The drawing under review shows one solid part. Ordinate dimensions are in mm from its lowest x, y, z. Give positions to 0.01 mm unless a question says otherwise; leave off trailing zeros. Order: outer loops, then holes, each group sorted by start corner. A loop starts at its lowest first (then second) coordinate and runs counter-clockwise, first axis right, second up. Notation, with made-up numbers: (-31.5, 80.25) -> (-3.5, 80.25) arc R12 cw to (-3.5, 93.25) -> close; hole circle Ø11 at (-15.75, -36). An arc over 180 degrees is marked (long way). One line per item, written item: value. Start each with the question number.
1) Consider section A-A (y = 0.4). State the section outline as (x, z) points.
2) For pin 1 (2.5 mm diameter, centred on x = 6.5, z = 8, fed in from -Y); pin 2 (6.5 mm diameter, centred on x = 34.5, z = 8, fed in from -Y), all flat-tipped, find the tip position at first contact; note any pin that passes through.
3) Consider section C-C (x = 6.5). State the section outline as (y, z) points, plus the area to 3 significant figures.
4) Consider section B-B (z = 8). State the section outline as (x, y) points.
5) Wall thickness on line 1 along X through (y, z) = (0.85, 8); line 2 along Z through (x, y) = (34.5, 0.85); line 3 along Z through (x, y) = (33.5, 1.7): over which ranges is each line inside the solid? List them lowest first. Write a range as from..to.
6) The part is to be moulded in two halves that separate along Y. For the marked faces 1 and 2, say which applies: released by +Y, released by -Y, zero draft, split by the parting line, or undercut.
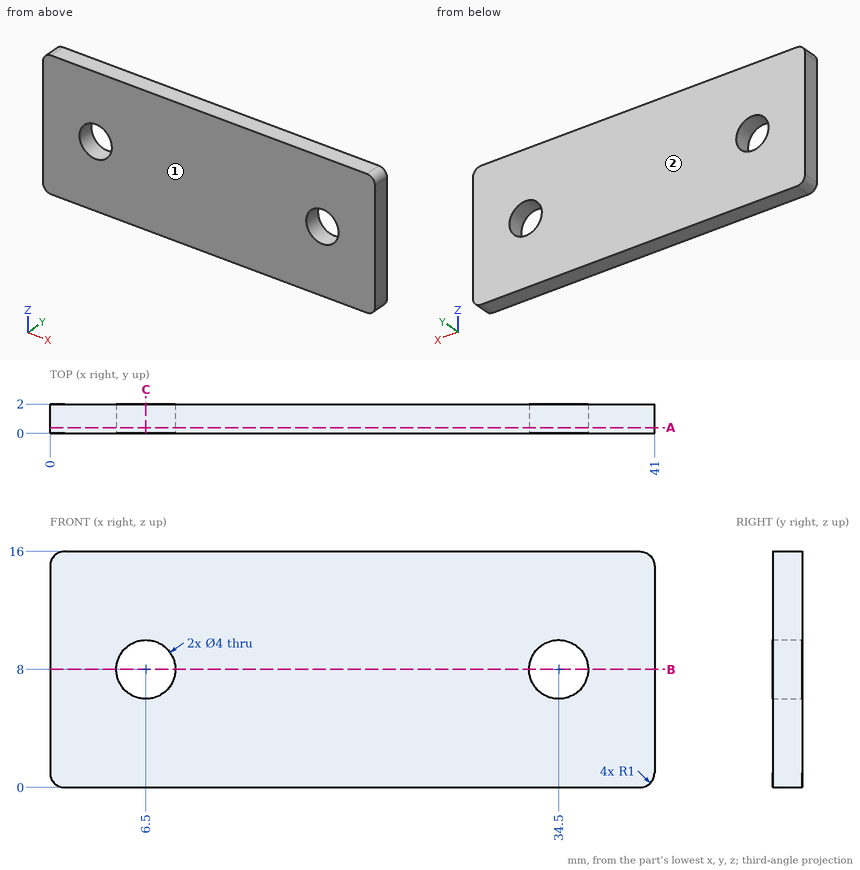
Checked values:
1. outline: (0, 1) arc R1 ccw to (1, 0) -> (40, 0) arc R1 ccw to (41, 1) -> (41, 15) arc R1 ccw to (40, 16) -> (1, 16) arc R1 ccw to (0, 15) -> close; hole circle Ø4 at (6.5, 8); hole circle Ø4 at (34.5, 8)
2. pin 1: passes through
2. pin 2: stops at y = 0
3. outline: (0, 0) -> (2, 0) -> (2, 6) -> (0, 6) -> close; (0, 10) -> (2, 10) -> (2, 16) -> (0, 16) -> close
3. area: 24.0 mm^2
4. outline: (0, 0) -> (4.5, 0) -> (4.5, 2) -> (0, 2) -> close; (8.5, 0) -> (32.5, 0) -> (32.5, 2) -> (8.5, 2) -> close; (36.5, 0) -> (41, 0) -> (41, 2) -> (36.5, 2) -> close
5. line 1: x = 0..4.5, 8.5..32.5, 36.5..41
5. line 2: z = 0..6, 10..16
5. line 3: z = 0..6.27, 9.73..16
6. face 1: released by -Y
6. face 2: released by +Y
